```python
from build123d import *

# Parameters (mm, degrees)
EXTRUDE_1_DEPTH     = 2
SKETCH_2_R          = 1.65
EXTRUDE_2_DEPTH     = 2.9
SKETCH_3_R          = 0.25
CUT_EXTRUDE_1_DEPTH = 10


with BuildPart() as part:
    # 草图1 → 凸台-拉伸1 (new body)
    with BuildSketch(Plane(origin=(0, 0, 0), x_dir=(1, 0, 0), z_dir=(0, 1, 0))):
        Polygon((-4.3, -1.074011537), (-1.074011537, -4.3), (1.074011537, -4.3), (4.3, -1.074011537), (4.3, 1.074011537), (1.074011537, 4.3), (-1.074011537, 4.3), (-4.3, 1.074011537), align=None)
    extrude(amount=EXTRUDE_1_DEPTH)

    # 草图2 → 凸台-拉伸2 (add)
    with BuildSketch(Plane(origin=(0, 2, 0), x_dir=(1, 0, 0), z_dir=(0, 1, 0))):
        with Locations(Location((0, 0, 0), (0, 0, 270))):
            Circle(SKETCH_2_R)
    extrude(amount=EXTRUDE_2_DEPTH)

    # 草图3 → 切除-拉伸1 (cut)
    with BuildSketch(Plane.XZ):
        with Locations(Location((0, 0, 0), (0, 0, 270))):
            Circle(SKETCH_3_R)
    extrude(amount=-CUT_EXTRUDE_1_DEPTH, mode=Mode.SUBTRACT)


solid = part.part
```
The listing builds one solid part. Answer for the finished solid, in the listing's coordinates (mm). A direction names the side the tool comes from. Give positions to 0.01 mm unless a question says otherwise; leave off trailing zeros. Loops run counter-clockwise (first coordinate to the right, second up) from the corner with the lowest first, then second, coordinate; pieces in that order, holes last. Notation, with made-up numbers: (0, 38) - (13, 38) arc R9 ccw to (13, 46) - close; hole circle Ø11 at (-8.5, 30.25). An arc over 180 degrees is marked (long way). Return JSON: item names as keys, results as strings. Group by question number.
1. Given pin 1 Ø4 at (x, z) = (-3, 2.5) entering from +Y, flat-ended and moving along its own axis, determine where the tip first touches the part or whether it passes through.
2. Straight lines are drawn through the part: line 1 (X direction, y = 2.5, z = 0); line 2 (Y direction, x = 0.25, z = 1.75); line 3 (Z direction, x = 2.5, y = 1.7). For each, find the intervals that lie inside material, in ascending order. Write a range as [from, to].
3. Find section A-A (z = 0). Write down the section's boundary in (x, y), then the cut area to 3 significant figures.
4. Find section C-C (x = 0). Write down the section's boundary in (y, z), then the cut area to 3 significant figures.
5. Find section D-D (y = 4.45). Write down the section's boundary in (x, z).
6. Which of the six approach directions +Z, -Z, +X, -X, +Y, -Y give full straight-line access (tool end or side, diameter ignored) to faces 1 (the flat face through (-2.664, 0.986, -2.71)), 2 (the cylindrical face through (-1, 3.43, -1.31))?
7. Find section B-B (y = 1.85). Write down the section's boundary in (x, z).
Verdict:
{
 "1": {"pin 1": "stops at y = 2"},
 "2": {"line 1": "x = [-1.65, -0.25], [0.25, 1.65]", "line 2": "y = [0, 2]", "line 3": "z = [-2.87, 2.87]"},
 "3": {"outline": "(-4.3, 0) - (-0.25, 0) - (-0.25, 4.9) - (-1.65, 4.9) - (-1.65, 2) - (-4.3, 2) - close; (0.25, 0) - (4.3, 0) - (4.3, 2) - (1.65, 2) - (1.65, 4.9) - (0.25, 4.9) - close", "area": "24.3 mm^2"},
 "4": {"outline": "(0, -4.3) - (2, -4.3) - (2, -1.65) - (4.9, -1.65) - (4.9, -0.25) - (0, -0.25) - close; (0, 0.25) - (4.9, 0.25) - (4.9, 1.65) - (2, 1.65) - (2, 4.3) - (0, 4.3) - close", "area": "24.3 mm^2"},
 "5": {"outline": "circle Ø3.3 at (0, 0); hole circle Ø0.5 at (0, 0)"},
 "6": {"face 1": "-Z, -X, +Y, -Y", "face 2": "+Y"},
 "7": {"outline": "(-4.3, -1.07) - (-1.07, -4.3) - (1.07, -4.3) - (4.3, -1.07) - (4.3, 1.07) - (1.07, 4.3) - (-1.07, 4.3) - (-4.3, 1.07) - close; hole circle Ø0.5 at (0, 0)"}
}
